For this review, take the finished solid that the model builds, in its own axes (mm). A direction names the side the tool comes from. Coordinates: 2 decimals unless noted, no trailing zeros. Loops run counter-clockwise (first coordinate to the right, second up) from the corner with the lowest first, then second, coordinate; pieces in that order, holes last. Notation, with made-up numbers: (78.25, -20.75) -> (132.25, -20.75) arc R25 cw to (132.25, 8.25) -> close; hole circle Ø1 at (83, 32). An arc over 180 degrees is marked (long way). Use a Markdown table: item, result.
from build123d import *

# Parameters (mm, degrees)
SKETCH1_R           = 2.1
BOSS_EXTRUDE1_DEPTH = 120


with BuildPart() as part:
    # Sketch1 → Boss-Extrude1 (new body, symmetric)
    with BuildSketch(Plane.XY):
        Polygon((5.499339828, 6.56), (3.59, 4.650660172), (-3.59, 4.650660172), (-5.499339828, 6.56), (-5.499339828, 8.2), (-3.1, 8.2), (-4.9, 10), (-10, 10), (-10, 4.9), (-8.2, 3.1), (-8.2, 5.499339828), (-6.56, 5.499339828), (-4.650660172, 3.59), (-4.650660172, -3.59), (-6.56, -5.499339828), (-8.2, -5.499339828), (-8.2, -3.1), (-10, -4.9), (-10, -10), (-4.9, -10), (-3.1, -8.2), (-5.499339828, -8.2), (-5.499339828, -6.56), (-3.59, -4.650660172), (3.59, -4.650660172), (5.499339828, -6.56), (5.499339828, -8.2), (3.1, -8.2), (4.9, -10), (10, -10), (10, -4.9), (8.2, -3.1), (8.2, -5.499339828), (6.56, -5.499339828), (4.650660172, -3.59), (4.650660172, 3.59), (6.56, 5.499339828), (8.2, 5.499339828), (8.2, 3.1), (10, 4.9), (10, 10), (4.9, 10), (3.1, 8.2), (5.499339828, 8.2), align=None)
        Circle(SKETCH1_R, mode=Mode.SUBTRACT)
    extrude(amount=BOSS_EXTRUDE1_DEPTH, both=True)


solid = part.part
(1) Mouldability with a two-part tool opening along Y and no side actions: class faces 3 (the face through (-7, 10, 2)), 4 (the face through (10, 7, 2)), 5 (the face through (4.651, 0, 2)), 6 (the face through (7, -10, 2)) as pulls with the +Y half, pulls with the -Y half, needs draft (parallel to the pull), parting line crosses it, or undercut.
Found:
| item | result |
|---|---|
| face 3 | pulls with the +Y half |
| face 4 | needs draft |
| face 5 | undercut |
| face 6 | pulls with the -Y half |
(2) For line 1 along Y through (x, z) = (0, 11.5); line 2 along X through (y, z) = (7.75, -73.5); line 3 along Y through (x, z) = (-5, -47), list the stretches that pass through material, from the lowest coordinate up.
Found:
| item | result |
|---|---|
| line 1 | y = -4.65 to -2.1, 2.1 to 4.65 |
| line 2 | x = -10 to -5.5, 5.5 to 10 |
| line 3 | y = -10 to -8.2, -6.06 to -3.94, 3.94 to 6.06, 8.2 to 10 |
(3) For faces 1 (the face through (-10, -7, 2)), 2 (the face through (0, 4.651, 2)), list the 3-axis set-ups (+Z, -Z, +X, -X, +Y, -Y) from which the entire face can be reached by the end or side of a thin tool; tool diameter is ignored.
Found:
| item | result |
|---|---|
| face 1 | +Z, -Z, -X, +Y, -Y |
| face 2 | +Z, -Z |
(4) For pin 1 Ø3.5 at (x, z) = (0.5, 1.5) entering from -Y; pin 2 Ø1.5 at (y, z) = (0.5, 34) entering from -X; pin 3 Ø5 at (x, z) = (-2.5, 3.5) entering from -Y; pin 4 Ø1.2 at (x, z) = (-4, 54) entering from -Y, all flat-tipped, find the tip position at first contact; note any pin that passes through.
Found:
| item | result |
|---|---|
| pin 1 | stops at y = -4.65 |
| pin 2 | stops at x = -4.65 |
| pin 3 | stops at y = -10 |
| pin 4 | stops at y = -9.7 |
(5) Take a section at A-A on y = 0. Write out the cut boundary in (x, z).
Found:
| item | result |
|---|---|
| outline | (-4.65, -120) -> (-2.1, -120) -> (-2.1, 120) -> (-4.65, 120) -> close; (2.1, -120) -> (4.65, -120) -> (4.65, 120) -> (2.1, 120) -> close |
